Could you check a few things on this drawing? It's one solid part, dimensions in mm from its lowest x, y, z. Give positions to 0.01 mm unless a question says otherwise; leave off trailing zeros. Order: outer loops, then holes, each group sorted by start corner. A loop starts at its lowest first (then second) coordinate and runs counter-clockwise, first axis right, second up.
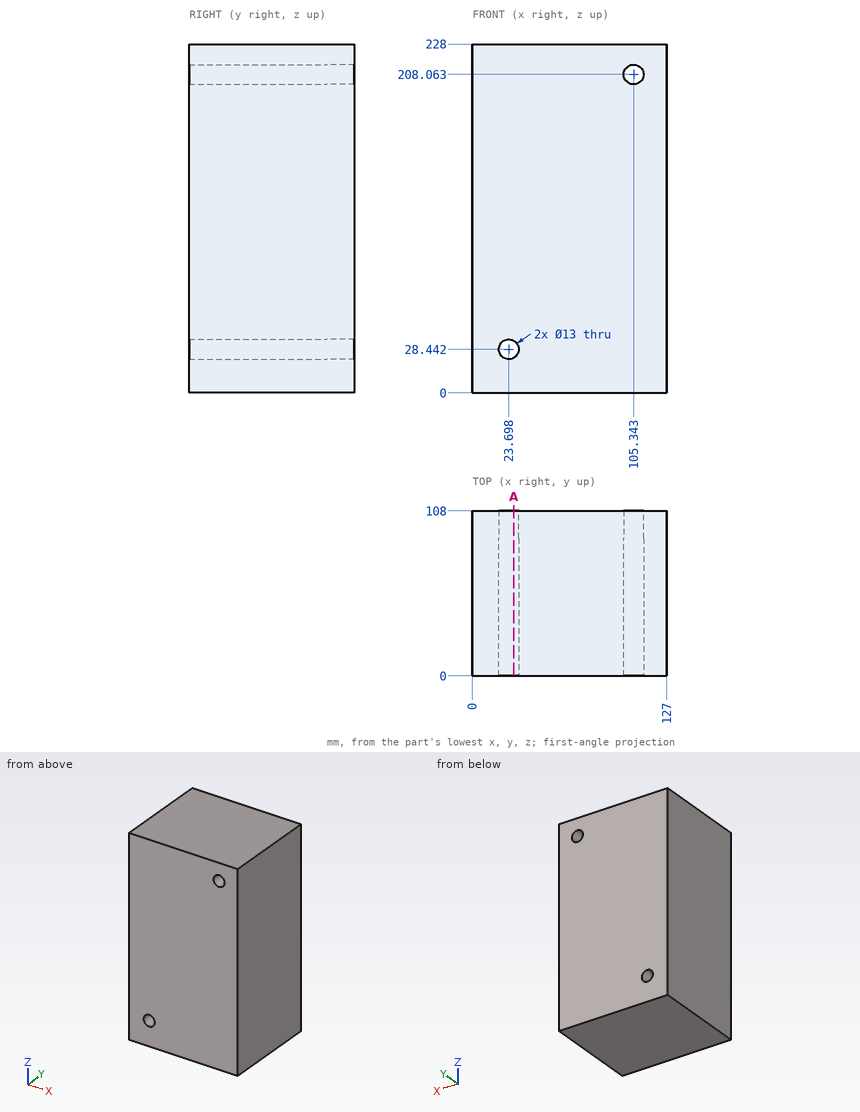
Item 1: Please list where these lines run through material, in increasing order: line 1 along X through (y, z) = (100.5, 22.5) (1 decimal); line 2 along Z through (x, y) = (29, 23.5) (1 decimal); line 3 along X through (y, z) = (38, 204) (1 decimal).
Findings:
line 1: x = 0 to 21.1, 26.3 to 127
line 2: z = 0 to 24.7, 32.2 to 228
line 3: x = 0 to 100.3, 110.4 to 127
Item 2: For pin 1 (1 mm diameter, centred on x = 67, y = 48, fed in from -Z), with a flat end and sliding along its axis, tell me the tip position at first contact or that it passes through.
Findings:
pin 1: stops at z = 0
Item 3: Imagine slicing it at A-A on x = 27. List the corners of the cut face in (y, z) for me, then the cut area to 3 significant figures.
Findings:
outline: (0, 0) - (108, 0) - (108, 22.84) - (0, 22.84) - close; (0, 34.04) - (108, 34.04) - (108, 228) - (0, 228) - close
area: 23,400 mm2
